Geometry: see drawing. Coordinates: mm, zero at the bounding-box minimum. A direction names the side the tool comes from. Give positions to 0.01 mm unless a question says otherwise; leave off trailing zeros. Write each loop counter-clockwise with the first axis right and the second up, starting at its lowest first coordinate (ties: lowest second). Pieces come first, ordered by that corner, then holes. Notation, with made-up numbers: M 82,-38.5 L 108,-38.5 A33 ccw 108,-9.5 Z; hole C -37.5,-3 d4. An arc over 180 degrees is marked long. Use a Markdown table: item, result. Add a question column.
1) Section A-A on z = 22.5. Return the cut outline in (x, y) (1 decimal), then the cut area to 3 significant figures.
2) Section B-B on z = 4. Return the cut outline in (x, y) (1 decimal), then the cut area to 3 significant figures.
3) Pin query (flat end, axial travel): pin 1 (6 mm diameter, centred on y = 60, z = 17.5, fed in from +X); pin 2 (5 mm diameter, centred on y = 13, z = 14.5, fed in from +X); pin 3 (4 mm diameter, centred on x = 8, z = 21, fed in from +Y). Return the tip coordinate at first contact, or that it passes through.
4) Draft query along X for the marked faces 3, 4 and 5. Return one class per face: +X half, -X half, draft (parallel to the pull), parting line (faces both ways), or undercut.
5) Set-up query: the marked faces 1 and 2. Return all of +Z, -Z, +X, -X, +Y, -Y with unobstructed straight access to the full face (end or side cutting, diameter ignored); none if empty.
6) Line query: line 1 (X direction, y = 43, z = 3); line 2 (X direction, y = 41, z = 16); line 3 (Y direction, x = 39, z = 6.5) (1 decimal). Output: solid intervals per line, ascending.
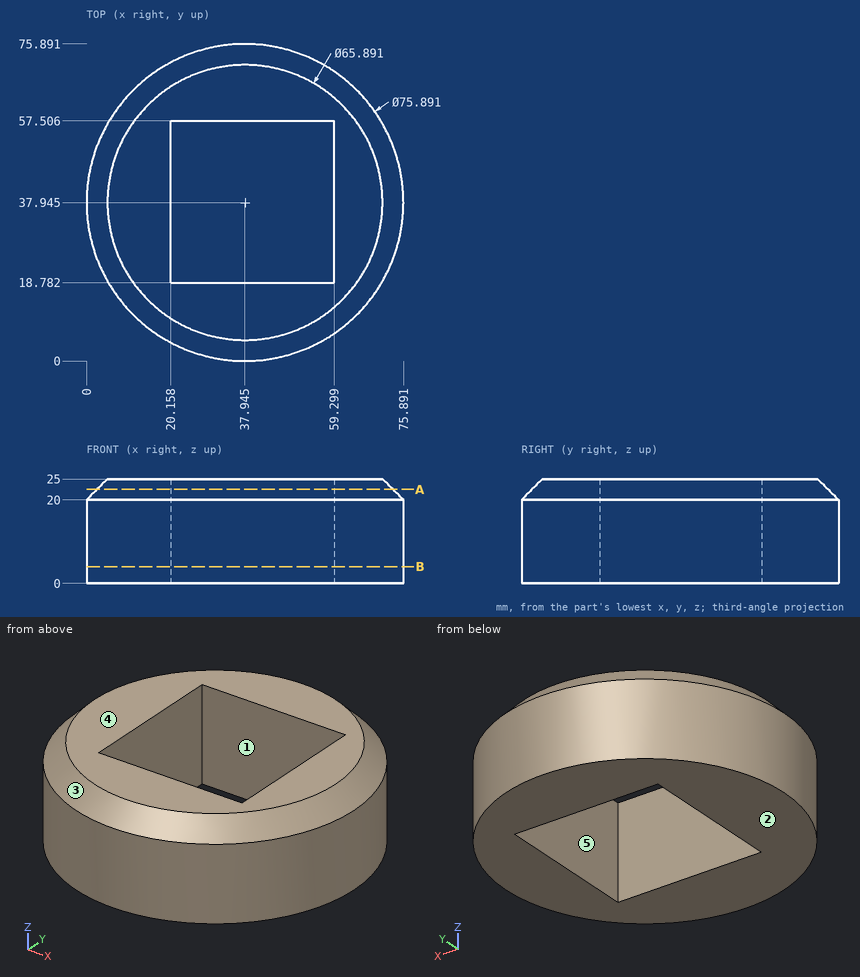
Found:
| question | item | result |
|---|---|---|
| 1 | outline | C 37.9,37.9 d70.9; hole M 20.2,18.8 L 59.3,18.8 L 59.3,57.5 L 20.2,57.5 Z |
| 1 | area | 2,430 mm² |
| 2 | outline | C 37.9,37.9 d75.9; hole M 20.2,18.8 L 59.3,18.8 L 59.3,57.5 L 20.2,57.5 Z |
| 2 | area | 3,010 mm² |
| 3 | pin 1 | x = 70.76 |
| 3 | pin 2 | x = 68.54 |
| 3 | pin 3 | y = 63.32 |
| 4 | face 3 | parting line |
| 4 | face 4 | draft |
| 4 | face 5 | undercut |
| 5 | face 1 | +Z, -Z |
| 5 | face 2 | -Z, +X, -X, +Y, -Y |
| 6 | line 1 | 0.34 to 20.16, 59.3 to 75.55 |
| 6 | line 2 | 0.12 to 20.16, 59.3 to 75.77 |
| 6 | line 3 | 0 to 18.8, 57.5 to 75.9 |
